Part model, mm, in its own coordinate system. A direction names the side the tool comes from. Round coordinates to 2 decimals unless told otherwise and drop trailing zeros. Order: outer loops, then holes, each group sorted by start corner. A loop starts at its lowest first (then second) coordinate and runs counter-clockwise, first axis right, second up. Notation, with made-up numbers: (2.25, 5) - (43.25, 5) arc R21 ccw to (43.25, 9) - close; hole circle Ø3 at (45, -38.75). An arc over 180 degrees is marked (long way). Answer as a JSON object with one key per item and string values.
```python
from build123d import *

# Parameters (mm, degrees)
SKETCH1_W                       = 450
SKETCH1_H                       = 20
BOSS_EXTRUDE1_DEPTH             = 14
SKETCH2_R                       = 10
CUT_EXTRUDE1_DEPTH              = 10
LPATTERN1_COUNT                 = 8
LPATTERN1_PITCH                 = 50
SKETCH3_R                       = 5
BOSS_EXTRUDE2_DEPTH             = 20
FILLET1_R                       = 14
BOSS_EXTRUDE3_REACH             = 472.315
BOSS_EXTRUDE4_REACH             = 247.603
BOSS_EXTRUDE4_DIRECTION_2_REACH = 247.603


with BuildPart() as part:
    # Sketch1 → Boss-Extrude1 (new, symmetric)
    with BuildSketch(Plane.XY):
        Rectangle(SKETCH1_W, SKETCH1_H)
    extrude(amount=BOSS_EXTRUDE1_DEPTH, both=True)

    # Sketch2 → Cut-Extrude1 (cut)
    with BuildSketch(Plane(origin=(0, 10, 0), x_dir=(1, 0, 0), z_dir=(0, 1, 0))):
        with Locations(Location((-175, 0, 0), (0, 0, 180))):
            Circle(SKETCH2_R)
    cut_extrude1 = extrude(amount=-CUT_EXTRUDE1_DEPTH, mode=Mode.SUBTRACT)

    # LPattern1: Cut-Extrude1 ×8
    with Locations(*[(i * LPATTERN1_PITCH, 0, 0) for i in range(1, LPATTERN1_COUNT)]):
        add(cut_extrude1, mode=Mode.SUBTRACT)

    # Sketch3 → Boss-Extrude2 (add)
    with BuildSketch(Plane(origin=(225, 0, 0), x_dir=(0, 0, -1), z_dir=(1, 0, 0))):
        with Locations((0, 4)):
            Circle(SKETCH3_R)
    boss_extrude2 = extrude(amount=BOSS_EXTRUDE2_DEPTH)

    # Mirror1: Boss-Extrude2 across plane
    add(boss_extrude2.mirror(Plane(origin=(0, 0, 0), x_dir=(0, 0, 1), z_dir=(1, 0, 0))))

    # Fillet1
    fillet1_edges = [part.edges().sort_by_distance(p)[0] for p in [
        (0, -10, 14),
        (0, -10, -14),
    ]]
    fillet(fillet1_edges, radius=FILLET1_R - 0.0001)  # a hair under: the kernel refuses the full size

    # Boss-Extrude3: up to this face of the body (flat: up to its plane)
    boss_extrude3_end = Plane(part.part.faces().sort_by_distance((225, 6.99995, -13.655906989))[0])
    # Sketch5 → Boss-Extrude3 (add, up to the picked face)
    with BuildSketch(Plane.ZY.offset(225), mode=Mode.PRIVATE) as boss_extrude3_sk1:
        Polygon((10, 0), (-10, 0), (-10, 5.358983849), align=None)
    boss_extrude3_tool1 = split(extrude(boss_extrude3_sk1.sketch, amount=-BOSS_EXTRUDE3_REACH, mode=Mode.PRIVATE), bisect_by=boss_extrude3_end, keep=Keep.BOTH, mode=Mode.PRIVATE)
    add(boss_extrude3_tool1.solids().sort_by(Axis((-225, 1.786328, -3.333333), (1, 0, 0)))[0])

    # Boss-Extrude4: up to this face of the body (flat: up to its plane)
    boss_extrude4_end = Plane(part.part.faces().sort_by_distance((-225, 6.99995, -13.655906989))[0])
    # Sketch6 → Boss-Extrude4 (add, up to the picked face)
    with BuildSketch(Plane(origin=(0, 0, 0), x_dir=(0, 0, -1), z_dir=(1, 0, 0)), mode=Mode.PRIVATE) as boss_extrude4_sk1:
        with BuildLine():
            Line((-19.5, 10), (-14, 10))
            Line((-14, 10), (-14, 4))
            ThreePointArc((-14, 4), (-9.899494937, -5.899494937), (0, -10))
            ThreePointArc((0, -10), (9.899494937, -5.899494937), (14, 4))
            Line((14, 4), (14, 10))
            Line((14, 10), (19.5, 10))
            Line((19.5, 10), (19.5, -15))
            Line((19.5, -15), (-13.829316686, -15))
            ThreePointArc((-13.829316686, -15), (-16.922455665, -12.305842336), (-19.5, -9.114877049))
            Line((-19.5, -9.114877049), (-19.5, 10))
        make_face()
    boss_extrude4_tool1 = split(extrude(boss_extrude4_sk1.sketch, amount=-BOSS_EXTRUDE4_REACH, mode=Mode.PRIVATE), bisect_by=boss_extrude4_end, keep=Keep.BOTH, mode=Mode.PRIVATE)
    add(boss_extrude4_tool1.solids().sort_by(Axis((0, 0.442561, 19.036751), (-1, 0, 0)))[0])

    # Boss-Extrude4 direction 2: up to this face of the body (flat: up to its plane)
    boss_extrude4_direction_2_end = Plane(part.part.faces().sort_by_distance((225, 6.99995, -13.655906989))[0])
    # Sketch6 → Boss-Extrude4 direction 2 (add, up to the picked face)
    with BuildSketch(Plane(origin=(0, 0, 0), x_dir=(0, 0, -1), z_dir=(1, 0, 0)), mode=Mode.PRIVATE) as boss_extrude4_direction_2_sk1:
        with BuildLine():
            Line((-19.5, 10), (-14, 10))
            Line((-14, 10), (-14, 4))
            ThreePointArc((-14, 4), (-9.899494937, -5.899494937), (0, -10))
            ThreePointArc((0, -10), (9.899494937, -5.899494937), (14, 4))
            Line((14, 4), (14, 10))
            Line((14, 10), (19.5, 10))
            Line((19.5, 10), (19.5, -15))
            Line((19.5, -15), (-13.829316686, -15))
            ThreePointArc((-13.829316686, -15), (-16.922455665, -12.305842336), (-19.5, -9.114877049))
            Line((-19.5, -9.114877049), (-19.5, 10))
        make_face()
    boss_extrude4_direction_2_tool1 = split(extrude(boss_extrude4_direction_2_sk1.sketch, amount=BOSS_EXTRUDE4_DIRECTION_2_REACH, mode=Mode.PRIVATE), bisect_by=boss_extrude4_direction_2_end, keep=Keep.BOTH, mode=Mode.PRIVATE)
    add(boss_extrude4_direction_2_tool1.solids().sort_by(Axis((0, 0.442561, 19.036751), (1, 0, 0)))[0])


solid = part.part
```
Item 1: Two-plate mould, pull along X, no slides. Class faces 4 (the flat face through (124.86, 2.717, -0.14)), 5 (the flat face through (245, 4, 0)), 6 (the cylindrical face through (234.86, -0.88, 1.08)), 7 (the flat face through (-225, -3, 0)): pulls with the +X half, pulls with the -X half, needs draft (parallel to the pull), parting line crosses it, or undercut.
Taken from the geometry:
{"face 4": "undercut", "face 5": "pulls with the +X half", "face 6": "needs draft", "face 7": "pulls with the -X half"}
Item 2: Tool access for faces 1 (the cylindrical face through (-234.86, -0.88, 1.08)), 2 (the flat face through (-3, 0, 19.5)), 3 (the cylindrical face through (76.302, 6.181, 9.915)): list every direction of +Z, -Z, +X, -X, +Y, -Y with a clear straight run to the whole face (end or side of a thin tool).
Taken from the geometry:
{"face 1": "-X", "face 2": "+Z, +X, -X, +Y, -Y", "face 3": "+Y"}
Item 3: Cut at A-A (x = 175). Write the cut outline in (y, z), plus the area to 3 significant figures.
Taken from the geometry:
{"outline": "(-15, -19.5) - (10, -19.5) - (10, -10) - (5.36, -10) - (0, 10) - (10, 10) - (10, 19.5) - (-9.11, 19.5) arc R23.5 ccw to (-15, 13.83) - close", "area": "814 mm2"}
Item 4: Probe L1, parallel to Z at x = -25, y = 7; L2, parallel to X at y = -1, z = 7.5; L3, parallel to Y at x = -80, z = 8.5. List the from-to ranges inside material, lowest first. Write a range as from..to.
Taken from the geometry:
{"L1": "-19.5..-10, 10..19.5", "L2": "-225..225", "L3": "-15..0.4"}
Item 5: Cut at B-B (x = -71). Write the cut outline in (y, z), plus the area to 3 significant figures.
Taken from the geometry:
{"outline": "(-15, -19.5) - (10, -19.5) - (10, -9.17) - (5.14, -9.17) - (0.22, 9.17) - (10, 9.17) - (10, 19.5) - (-9.11, 19.5) arc R23.5 ccw to (-15, 13.83) - close", "area": "826 mm2"}
Item 6: Drop flat-ended pins along their axis: P1, Ø16, axis at x = 75, z = 0, coming from the +Y side; P2, Ø1, axis at x = 70.5, y = -11, coming from the +Z side; P3, Ø18, axis at x = 25, z = 0, coming from the +Y side. Give the stop position or say it passes through.
Taken from the geometry:
{"P1": "y = 4.82", "P2": "z = 18.49", "P3": "y = 5.09"}
